```python
from build123d import *

# Parameters (mm, degrees)
SKETCH1_R           = 15
BOSS_EXTRUDE1_DEPTH = 20
SKETCH2_W           = 50
SKETCH2_H           = 10
CUT_EXTRUDE1_DEPTH  = 84
SKETCH3_R           = 5.297885383
CUT_EXTRUDE2_DEPTH  = 20
SKETCH4_W           = 30.252743008
SKETCH4_H           = 4.249478602
CUT_EXTRUDE3_DEPTH  = 31


with BuildPart() as part:
    # Sketch1 → Boss-Extrude1 (new body)
    with BuildSketch(Plane.XY):
        with BuildLine():
            Line((-72.1, -25), (72.1, -25))
            ThreePointArc((72.1, -25), (114.77766953, -42.67766953), (97.1, 0))
            Line((97.1, 0), (-97.1, 0))
            ThreePointArc((-97.1, 0), (-114.77766953, -42.67766953), (-72.1, -25))
        make_face()
        with Locations((-97.1, -25)):
            Circle(SKETCH1_R, mode=Mode.SUBTRACT)
        with Locations((97.1, -25)):
            Circle(SKETCH1_R, mode=Mode.SUBTRACT)
    extrude(amount=BOSS_EXTRUDE1_DEPTH)

    # Sketch2 → Cut-Extrude1 (cut)
    with BuildSketch(Plane(origin=(0, 0, 0), x_dir=(1, 0, 0), z_dir=(0, 1, 0))):
        with Locations((97.1, -5)):
            Rectangle(SKETCH2_W, SKETCH2_H)
        with Locations((-97.1, -15)):
            Rectangle(SKETCH2_W, SKETCH2_H)
    extrude(amount=-CUT_EXTRUDE1_DEPTH, mode=Mode.SUBTRACT)

    # Sketch3 → Cut-Extrude2 (cut)
    with BuildSketch(Plane.XY.offset(20)):
        with Locations((-54.754964617, -12.5)):
            Circle(SKETCH3_R)
        with Locations((54.754964617, -12.5)):
            Circle(SKETCH3_R)
    extrude(amount=-CUT_EXTRUDE2_DEPTH, mode=Mode.SUBTRACT)

    # Sketch4 → Cut-Extrude3 (cut)
    with BuildSketch(Plane(origin=(0, 0, 0), x_dir=(1, 0, 0), z_dir=(0, 1, 0))):
        with Locations((-15.126371504, -17.875260699)):
            Rectangle(SKETCH4_W, SKETCH4_H)
        with Locations((15.126371504, -2.124739301)):
            Rectangle(SKETCH4_W, SKETCH4_H)
    extrude(amount=-CUT_EXTRUDE3_DEPTH, mode=Mode.SUBTRACT)


solid = part.part
```
Can you work these out from the model? Positions are in its coordinate system, mm. A direction names the side the tool comes from. Give positions to 0.01 mm unless a question says otherwise; leave off trailing zeros. Write each loop counter-clockwise with the first axis right and the second up, starting at its lowest first coordinate (ties: lowest second). Pieces come first, ordered by that corner, then holes. Notation, with made-up numbers: (19.25, 63) -> (53.25, 63) arc R20 ccw to (53.25, 80) -> close; hole circle Ø2 at (6.25, 29). An arc over 180 degrees is marked (long way). Write item = value, one per line.
(1) Suppose I cut it at A-A on z = 12.5. Write out the boundary of the cut face in (x, y).
Worked out:
outline = (-72.1, -25) -> (72.1, -25) arc R25 ccw (long way) to (97.1, 0) -> (-72.1, 0) -> close; hole circle Ø10.6 at (-54.75, -12.5); hole circle Ø10.6 at (54.75, -12.5); hole circle Ø30 at (97.1, -25)
(2) Suppose I cut it at D-D on x = 38. Write out the boundary of the cut face in (y, z), then the cut area to 3 significant figures.
Worked out:
outline = (-25, 0) -> (0, 0) -> (0, 20) -> (-25, 20) -> close
area = 500 mm^2
(3) I'm going to push flat-ended pins straight in: P1, Ø7.5, axis at x = -8.5, y = -8.5, coming from the +Z side; P2, Ø3.5, axis at y = -14.5, z = 18.5, coming from the -X side; P3, Ø15, axis at x = -88, y = -29.5, coming from the +Z side. Where does each tip first touch, or does it pass through?
Worked out:
P1 = 15.75
P2 = -72.1
P3 = 10
(4) I need wall thicknesses on probe 1 along Y at (x, z) = (-97.1, 6.25); probe 2 along Y at (x, z) = (71, 5.25); probe 3 along X at (y, z) = (-29, 17.75). Which ranges of each line are inside material? Lowest first, please. Write a range as from..to.
Worked out:
probe_1 = -50..-40, -10..0
probe_2 = -25..0
probe_3 = 72.42..82.64, 111.56..121.78
(5) Thinking about a two-plate mould opening in X: for faces 1 (the face through (-58.96, -15.72, 10.14)), 2 (the face through (1, 0, 10)), 3 (the face through (-72.1, -12, 15)), which applies, released by +X, released by -X, zero draft, split by the parting line, or undercut?
Worked out:
face_1 = undercut
face_2 = zero draft
face_3 = released by -X
(6) Suppose I cut it at C-C on x = -102. Write out the boundary of the cut face in (y, z), then the cut area to 3 significant figures.
Worked out:
outline = (-49.52, 0) -> (-39.18, 0) -> (-39.18, 10) -> (-49.52, 10) -> close; (-10.82, 0) -> (-0.48, 0) -> (-0.48, 10) -> (-10.82, 10) -> close
area = 207 mm^2
(7) For faces 4 (the face through (0, -12, 18)), 5 (the face through (30.253, -12, 2)), 6 (the face through (-1, -25, 10)), 7 (the face through (86, -14, 10)), which set-ups out of +Z, -Z, +X, -X, +Y, -Y let a thin tool reach every point of the face, with its end or its side?
Worked out:
face_4 = +Z, +Y, -Y
face_5 = -Z, +Y, -Y
face_6 = +Z, -Z, -Y
face_7 = -Z, +X, +Y, -Y
(8) Suppose I cut it at B-B on y = -28.5. Write out the boundary of the cut face in (x, z).
Worked out:
outline = (-121.85, 0) -> (-111.69, 0) -> (-111.69, 10) -> (-121.85, 10) -> close; (-82.51, 0) -> (-72.35, 0) -> (-72.35, 10) -> (-82.51, 10) -> close; (72.35, 10) -> (82.51, 10) -> (82.51, 20) -> (72.35, 20) -> close; (111.69, 10) -> (121.85, 10) -> (121.85, 20) -> (111.69, 20) -> close
